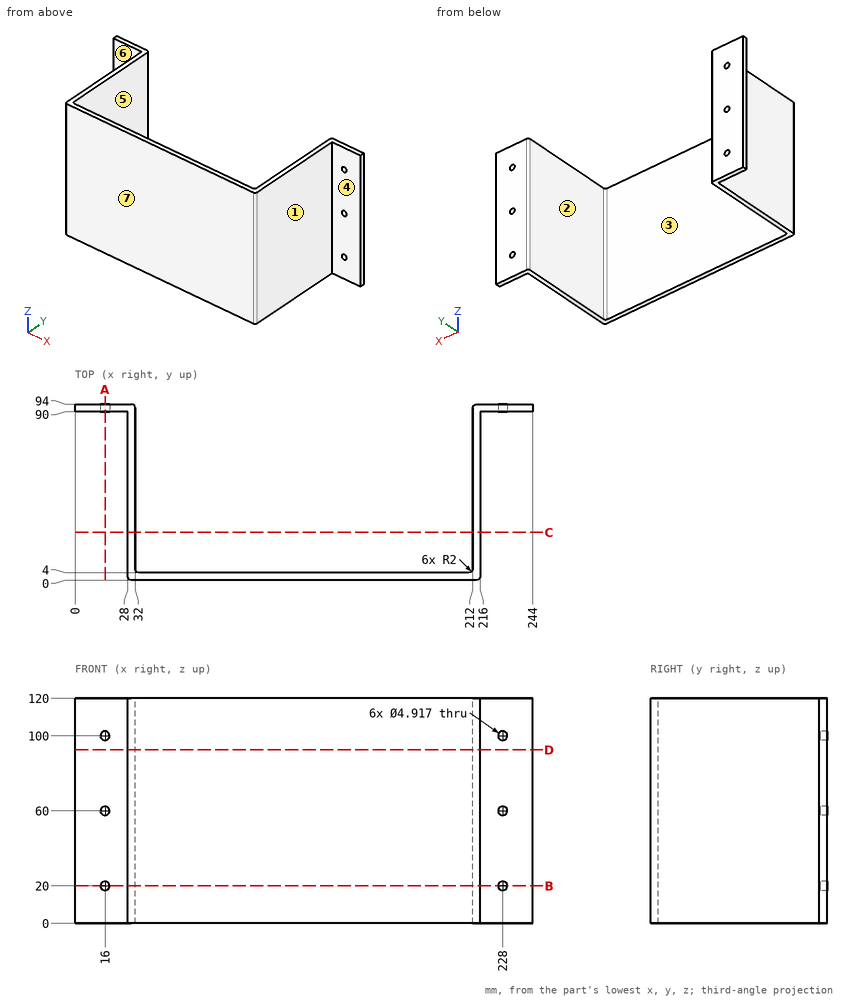
The figure shows three views and two pictorial views of one solid part (mm, origin at its lowest corner). Answer the questions. A direction names the side the tool comes from. Give positions to 0.01 mm unless a question says otherwise; leave off trailing zeros. Write each loop counter-clockwise with the first axis right and the second up, starting at its lowest first coordinate (ties: lowest second). Pieces come first, ordered by that corner, then holes. Notation, with made-up numbers: (-9, 9) -> (49, 9) arc R18 ccw to (49, 21) -> close; hole circle Ø9 at (32.5, 69.25). An arc over 180 degrees is marked (long way). Answer as a JSON object with one key per item and string values.
1) Flat-ended cylindrical pins translate along their axes: pin 1 Ø22.5 at (x, z) = (8.5, 68.5) entering from -Y; pin 2 Ø2 at (x, z) = (186, 68) entering from +Y; pin 3 Ø4 at (y, z) = (29, 36.5) entering from +X. Find the tip coordinate at first contact, or state that the pin passes through.
Findings below:
{"pin 1": "stops at y = 90", "pin 2": "stops at y = 4", "pin 3": "stops at x = 216"}
2) A tool of negligible diameter and unlimited length cuts with its end or side. For the marked faces 5, 6 and 7, from which of +Z, -Z, +X, -X, +Y, -Y can it reach the whole face along a straight path? Write none if from no direction.
Findings below:
{"face 5": "+Z, -Z, +Y", "face 6": "+Z, -Z, -X, -Y", "face 7": "+Z, -Z, +X, -X, -Y"}
3) Section B-B on z = 20 is taken. Write down the section's boundary in (x, y).
Findings below:
{"outline": "(0, 90) -> (13.54, 90) -> (13.54, 94) -> (0, 94) -> close; (18.46, 90) -> (28, 90) -> (28, 2) arc R2 ccw to (30, 0) -> (214, 0) arc R2 ccw to (216, 2) -> (216, 90) -> (225.54, 90) -> (225.54, 94) -> (214, 94) arc R2 ccw to (212, 92) -> (212, 6) arc R2 cw to (210, 4) -> (34, 4) arc R2 cw to (32, 6) -> (32, 92) arc R2 ccw to (30, 94) -> (18.46, 94) -> close; (230.46, 90) -> (244, 90) -> (244, 94) -> (230.46, 94) -> close"}
4) Section D-D on z = 92.5 is taken. Write down the section's boundary in (x, y), then the cut area to 3 significant figures.
Findings below:
{"outline": "(0, 90) -> (28, 90) -> (28, 2) arc R2 ccw to (30, 0) -> (214, 0) arc R2 ccw to (216, 2) -> (216, 90) -> (244, 90) -> (244, 94) -> (214, 94) arc R2 ccw to (212, 92) -> (212, 6) arc R2 cw to (210, 4) -> (34, 4) arc R2 cw to (32, 6) -> (32, 92) arc R2 ccw to (30, 94) -> (0, 94) -> close", "area": "1,690 mm^2"}
5) Section C-C on y = 25.5 is taken. Write down the section's boundary in (x, z), then the cut area to 3 significant figures.
Findings below:
{"outline": "(28, 0) -> (32, 0) -> (32, 120) -> (28, 120) -> close; (212, 0) -> (216, 0) -> (216, 120) -> (212, 120) -> close", "area": "960 mm^2"}
6) Section A-A on x = 16 is taken. Write down the section's boundary in (y, z), then the cut area to 3 significant figures.
Findings below:
{"outline": "(90, 0) -> (94, 0) -> (94, 17.54) -> (90, 17.54) -> close; (90, 22.46) -> (94, 22.46) -> (94, 57.54) -> (90, 57.54) -> close; (90, 62.46) -> (94, 62.46) -> (94, 97.54) -> (90, 97.54) -> close; (90, 102.46) -> (94, 102.46) -> (94, 120) -> (90, 120) -> close", "area": "421 mm^2"}
7) For a pull along X with two mould halves and no side action, classify the marked faces 1, 2, 3 and 4 as pulls with the +X half, pulls with the -X half, needs draft (parallel to the pull), parting line crosses it, or undercut.
Findings below:
{"face 1": "pulls with the +X half", "face 2": "undercut", "face 3": "undercut", "face 4": "needs draft"}
8) Straight lines are drawn through the part: probe 1 along X at (y, z) = (92, 100); probe 2 along Z at (x, y) = (16, 92); probe 3 along X at (y, z) = (19.5, 10). For each, find the intervals that lie inside material, in ascending order. Write a range as from..to.
Findings below:
{"probe 1": "x = 0..13.54, 18.46..32, 212..225.54, 230.46..244", "probe 2": "z = 0..17.54, 22.46..57.54, 62.46..97.54, 102.46..120", "probe 3": "x = 28..32, 212..216"}
